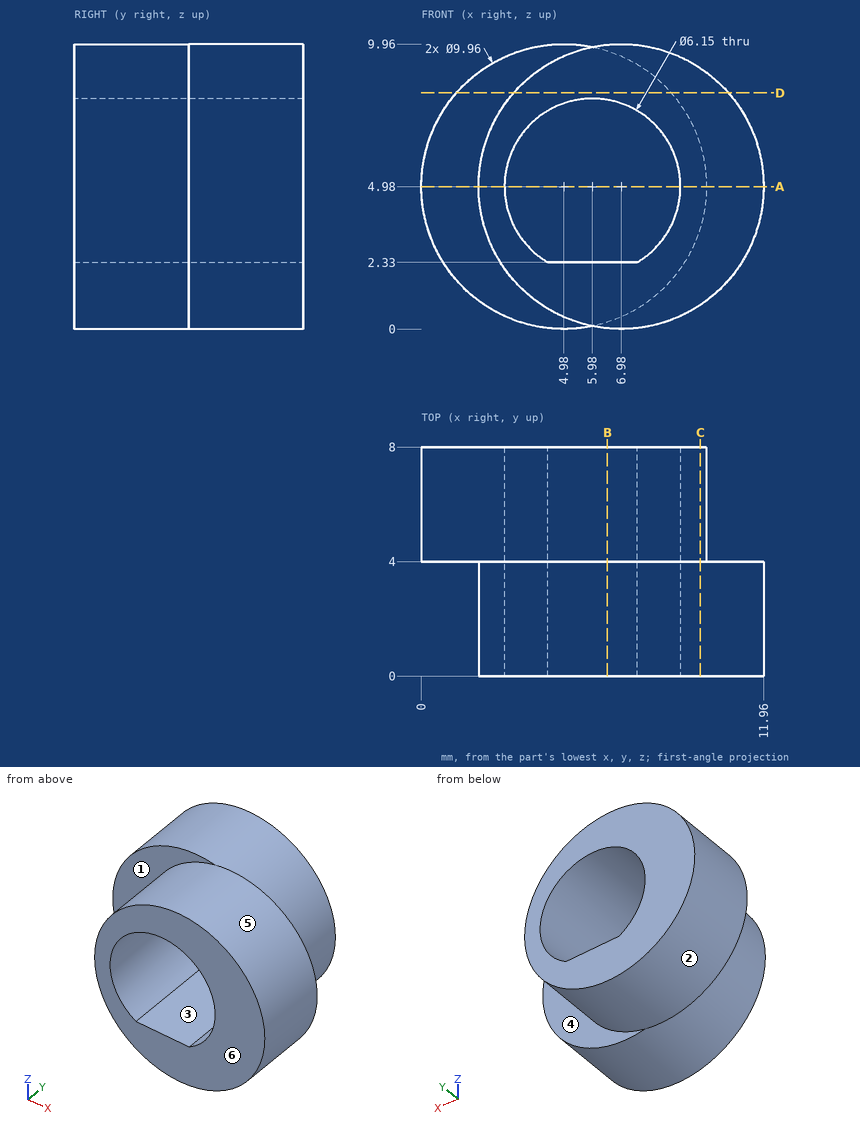
Geometry: see drawing. Coordinates: mm, zero at the bounding-box minimum. A direction names the side the tool comes from. Round coordinates to 2 decimals unless told otherwise and drop trailing zeros. Write each loop counter-clockwise with the first axis right and the second up, starting at its lowest first coordinate (ties: lowest second). Pieces come first, ordered by that corner, then holes. Notation, with made-up numbers: M 69.25,-30.5 L 101.25,-30.5 A21 cw 101.25,-12.5 Z; hole C 27.5,83 d6. An arc over 180 degrees is marked long. Answer as a JSON object with one key per item and string values. Group by question number.
(1) First-contact query: pin 1 (5 mm diameter, centred on x = 4, z = 6, fed in from -Y); pin 2 (2 mm diameter, centred on y = 4, z = 8.5, fed in from -X). Flat tips, straight axial feed; report the tip coordinate or a pass-through.
(2) Ray query, line 1 (X direction, y = 5, z = 4.98) (3 decimals); line 2 (X direction, y = 2, z = 4.98) (3 decimals); line 3 (Y direction, x = 2.75, z = 8.75). Return the intervals inside material, ascending. Write a range as [from, to].
(3) Mould query, pull axis X, two halves, no side actions, for the marked faces 1, 2 and 3. Classes: +X half, -X half, draft (parallel to the pull), parting line (faces both ways), or undercut.
(4) Reachability of the marked faces 4, 5 and 6 from +Z, -Z, +X, -X, +Y, -Y: full face, straight path, thin tool, end or side. Return the list, or none.
(5) Section query B-B on x = 6.5. Output: boundary loops of the cut face in (y, z), then the cut area to 3 significant figures.
(6) Section query A-A on z = 4.98. Output: boundary loops of the cut face in (x, y) (3 decimals).
(7) Section query D-D on z = 8.25. Output: boundary loops of the cut face in (x, y).
(8) Section query C-C on x = 9.75. Output: boundary loops of the cut face in (y, z), then the cut area to 3 significant figures.
Computed values:
{
 "1": {"pin 1": "y = 0", "pin 2": "x = 0.68"},
 "2": {"line 1": "[0, 2.905], [9.055, 9.96]", "line 2": "[2, 2.905], [9.055, 11.96]", "line 3": "[4, 8]"},
 "3": {"face 1": "draft", "face 2": "parting line", "face 3": "undercut"},
 "4": {"face 4": "+X, +Y", "face 5": "-Y", "face 6": "+Z, -Z, +X, -X, -Y"},
 "5": {"outline": "M 0,0.02 L 4,0.02 L 4,0.24 L 8,0.24 L 8,2.33 L 0,2.33 Z; M 0,8.01 L 8,8.01 L 8,9.72 L 4,9.72 L 4,9.94 L 0,9.94 Z", "area": "32.1 mm^2"},
 "6": {"outline": "M 0,4 L 2,4 L 2,0 L 2.905,0 L 2.905,8 L 0,8 Z; M 9.055,0 L 11.96,0 L 11.96,4 L 9.96,4 L 9.96,8 L 9.055,8 Z"},
 "7": {"outline": "M 1.22,4 L 3.22,4 L 3.22,0 L 10.74,0 L 10.74,4 L 8.74,4 L 8.74,8 L 1.22,8 Z"},
 "8": {"outline": "M 0,0.84 L 4,0.84 L 4,3.55 L 8,3.55 L 8,6.41 L 4,6.41 L 4,9.12 L 0,9.12 Z", "area": "44.6 mm^2"}
}
